Autodesk Inventor part; units mm, degrees
ref_plane "YZ Plane" through (0, 0, 0) normal (1, 0, 0) x (0, 1, 0)
ref_plane "XZ Plane" through (0, 0, 0) normal (0, 1, 0) x (-1, 0, 0)
ref_plane "XY Plane" through (0, 0, 0) normal (0, 0, 1) x (1, 0, 0)
sketch "Sketch1" plane through (0, 0, 0) normal (0, 0, 1) x (1, 0, 0)
  circle A0 centre (0, 0) radius 2.7
  dimension "d0" = 5.4
extrude "Extrusion1" add sketch "Sketch1" along normal blind 3.7
sketch "Sketch2" plane through (0, 0, 3.7) normal (0, 0, 1) x (1, 0, 0)
  circle A0 centre (0, 0) radius 1.27
  circle A1 centre (1.27, 0) radius 0.215
  circle A2 centre (0, 1.27) radius 0.215
  circle A3 centre (-1.27, 0) radius 0.215
  circle A4 centre (0, -1.27) radius 0.215
  dimension "d3" = 2.54
  dimension "d4" = 0.43
  dimension "d7" = 360
extrude "Extrusion2" add sketch "Sketch2" along normal blind 12.7 contours A0 A1 | A0 A1 | A2 A0 | A0 A2 | A4 A0 | A0 A4 | A3 A0 | A0 A3
sketch "Sketch3" plane through (0, 0, 3.7) normal (0, 0, 1) x (1, 0, 0)
  line L0 (2.9561, -2.2765) -> (2.249, -2.9836)
  line L1 (2.249, -2.9836) -> (1.4633, -2.1979)
  line L2 (1.4633, -2.1979) -> (2.1704, -1.4908)
  line L3 (2.1704, -1.4908) -> (2.9561, -2.2765)
  circle A0 centre (0, 0) radius 2.7
  point P0 (2.2185, -1.5389)
  point P1 (1.5062, -2.2408)
  dimension "d11" = 1
  dimension "d12" = 6.4
extrude "Extrusion3" add sketch "Sketch3" along normal blind 0.2
sketch "Sketch4" plane through (0, 0, 3.9) normal (0, 0, 1) x (1, 0, 0)
  line L0 (-0.2098, -1.6461) -> (0.1759, -1.6461) construction
  line L1 (0.1759, -1.6461) -> (0.1759, -2.1461) construction
  line L2 (0.1759, -2.1461) -> (-0.2098, -2.1461) construction
  line L3 (-0.2098, -2.1461) -> (-0.2098, -1.6461) construction
  line L4 (1.5616, 0.2129) -> (1.9473, 0.2129) construction
  line L5 (1.9473, 0.2129) -> (1.9473, -0.2871) construction
  line L6 (1.9473, -0.2871) -> (1.5616, -0.2871) construction
  line L7 (1.5616, -0.2871) -> (1.5616, 0.2129) construction
  line L8 (-1.9384, 0.2505) -> (-1.5527, 0.2505) construction
  line L9 (-1.5527, 0.2505) -> (-1.5527, -0.2495) construction
  line L10 (-1.5527, -0.2495) -> (-1.9384, -0.2495) construction
  line L11 (-1.9384, -0.2495) -> (-1.9384, 0.2505) construction
  line L12 (-0.1933, 2.1269) -> (0.1924, 2.1269) construction
  line L13 (0.1924, 2.1269) -> (0.1924, 1.6269) construction
  line L14 (0.1924, 1.6269) -> (-0.1933, 1.6269) construction
  line L15 (-0.1933, 1.6269) -> (-0.1933, 2.1269) construction
  point P0 (0, 0)
move faces "Move1" translate (0, 0, -10) faces at (-0.0635, 1.2367, 16.4) (1.2786, 0.0711, 16.4) (-0.0635, -1.3033, 16.4) (-1.2446, 0.067, 16.4)
move faces "Move2" translate (0, 0, 1.588) faces at (-1.2446, 0.067, 6.4) (-0.0635, 1.2367, 6.4) (1.2786, 0.0711, 6.4) (-0.0635, -1.3033, 6.4)
properties part number "Sensor"
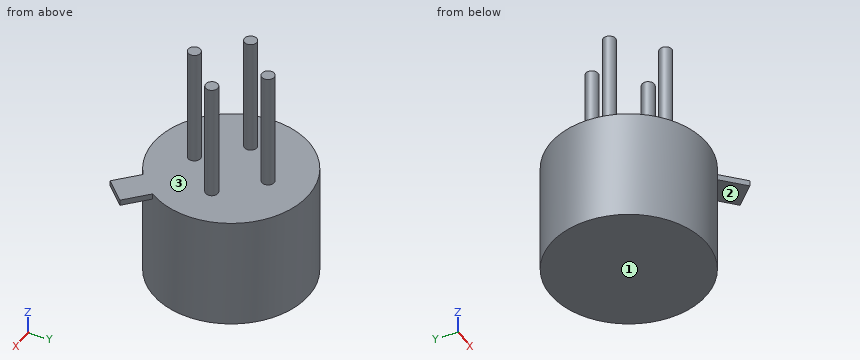
Part model, mm, in its own coordinate system. Face numbers are marked on the shaded views. A direction names the side the tool comes from. Round coordinates to 2 decimals unless told otherwise and drop trailing zeros. Write each loop counter-clockwise with the first axis right and the second up, starting at its lowest first coordinate (ties: lowest second). Pieces come first, ordered by that corner, then holes.
Item 1: Cut at A-A, the plane z = 7.25. Give the cut face in (x, y) (3 decimals), plus the area to 3 significant figures.
Results:
outline: circle Ø0.43 at (-1.27, 0); circle Ø0.43 at (0, -1.27); circle Ø0.43 at (0, 1.27); circle Ø0.43 at (1.27, 0)
area: 0.581 mm2
Item 2: Which spindle directions (+Z, -Z, +X, -X, +Y, -Y) get a long thin tool onto all of the face, cutting with end or side? Do the marked faces 1, 2 and 3. Say none if no direction does.
Results:
face 1: -Z, +X, -X, +Y, -Y
face 2: -Z, +X, -Y
face 3: +Z
Item 3: Drop flat-ended pins along their axis: pin 1 Ø1.5 at (x, y) = (0, -1.5) entering from -Z; pin 2 Ø1.5 at (y, z) = (-0.5, 2.5) entering from +X; pin 3 Ø2 at (x, z) = (-0.5, 6) entering from -Y (3 decimals). Give the stop position or say it passes through.
Results:
pin 1: stops at z = 0
pin 2: stops at x = 2.7
pin 3: stops at y = -1.485
Item 4: Probe L1, parallel to Z at x = 2.3, y = -0.8; L2, parallel to Y at x = 1.95, z = 2.25; L3, parallel to Y at x = -0.1, z = 7.5. List the from-to ranges inside material, lowest first.
Results:
L1: z = 0 to 3.9
L2: y = -1.87 to 1.87
L3: y = -1.46 to -1.08, 1.08 to 1.46
Item 5: Cut at B-B, the plane z = 2. Give the cut face in (x, y).
Results:
outline: circle Ø5.4 at (0, 0)
